from build123d import *

# Parameters (mm, degrees)
SKETCH1_R           = 1.5
BOSS_EXTRUDE1_DEPTH = 5


with BuildPart() as part:
    # Sketch1 → Boss-Extrude1 (new body)
    with BuildSketch(Plane(origin=(0, 0, 0), x_dir=(1, 0, 0), z_dir=(0, 1, 0))):
        with BuildLine():
            Line((12.5, -22.5), (-12.5, -22.5))
            ThreePointArc((-12.5, -22.5), (-19.571067812, -19.571067812), (-22.5, -12.5))
            Line((-22.5, -12.5), (-22.5, 12.5))
            ThreePointArc((-22.5, 12.5), (-19.571067812, 19.571067812), (-12.5, 22.5))
            Line((-12.5, 22.5), (12.5, 22.5))
            ThreePointArc((12.5, 22.5), (19.571067812, 19.571067812), (22.5, 12.5))
            Line((22.5, 12.5), (22.5, -12.5))
            ThreePointArc((22.5, -12.5), (19.571067812, -19.571067812), (12.5, -22.5))
        make_face()
        with Locations(Location((-15, 15, 0), (0, 0, 270))):
            Circle(SKETCH1_R, mode=Mode.SUBTRACT)
        with Locations(Location((15, 15, 0), (0, 0, 90))):
            Circle(SKETCH1_R, mode=Mode.SUBTRACT)
        with Locations(Location((15, -15, 0), (0, 0, 270))):
            Circle(SKETCH1_R, mode=Mode.SUBTRACT)
        with Locations(Location((-15, -15, 0), (0, 0, 90))):
            Circle(SKETCH1_R, mode=Mode.SUBTRACT)
    extrude(amount=BOSS_EXTRUDE1_DEPTH)

    # Sketch5 → Revolve5 (revolve)
    with BuildSketch(Plane.XY, mode=Mode.PRIVATE) as revolve5_sk:
        with BuildLine():
            Line((0, 0), (0, -30))
            Line((0, -30), (-14.490872109, -30))
            ThreePointArc((-14.490872109, -30), (-10.310219401, -15), (-14.490872109, 0))
            Line((-14.490872109, 0), (0, 0))
        make_face()
    revolve(revolve5_sk.sketch.rotate(Axis((0, 6.623218914, 0), (0, -1, 0)), 270), axis=Axis((0, 6.623218914, 0), (0, -1, 0)))

    # Sketch6 → Revolve6 (revolve)
    with BuildSketch(Plane(origin=(0, 0, 0), x_dir=(0, 0, -1), z_dir=(1, 0, 0))):
        with BuildLine():
            Line((0, -17.323751058), (0, -59.119175033))
            ThreePointArc((0, -59.119175033), (-20.897711988, -38.221463045), (0, -17.323751058))
        make_face()
    revolve(axis=Axis((0, -62.962580504, 0), (0, 1, 0)))


solid = part.part
CAD build for the part. Positions are in the model's coordinates, mm. A direction names the side the tool comes from. Round coordinates to 2 decimals unless told otherwise and drop trailing zeros. Write each loop counter-clockwise with the first axis right and the second up, starting at its lowest first coordinate (ties: lowest second). Pieces come first, ordered by that corner, then holes. Notation, with made-up numbers: M 29.25,69.25 L 62.25,69.25 A21 ccw 62.25,98.25 Z; hole C -0.5,24.5 d9. An arc over 180 degrees is marked long. Use a Markdown table: item, result. Add a question column.
1. Flat gauge pins, fed straight in: P1, Ø10, axis at y = -45, z = 1, coming from the +X side; P2, Ø12, axis at y = -31, z = -15.5, coming from the -X side; P3, Ø6, axis at x = 1, z = -8, coming from the -Y side. Where does each tip first touch, or does it go through?
2. Pull direction X, two halves, no side cores. Call faces 4 (the face through (14.93, 2.46, -13.5)), 5 (the face through (19.65, 2.46, 19.49)), 6 (the face through (-19.65, 2.46, -19.49)), 7 (the face through (-15.07, 2.46, 16.5)): released by +X, released by -X, zero draft, split by the parting line, or undercut.
3. Slice it at B-B on y = -49.5. Give the cut face in (x, z).
4. Slice it at A-A on y = -15.5. Give the cut face in (x, z), then the cut area to 3 significant figures.
5. 3-axis set-ups, long thin cutter, end or side, ignore diameter. For faces 1 (the face through (0, 2, 22.5)), 2 (the face through (0, 0, -15)), 3 (the face through (15.07, 2.46, 13.5)): which of +Z, -Z, +X, -X, +Y, -Y reach the whole face in a straight line?
6. Drill centre lines: probe 1 along X at (y, z) = (2, -15); probe 2 along Y at (x, z) = (16, -16.5); probe 3 along Y at (x, z) = (16.5, 3). Where is each one in solid material? Low to high.
Reply:
| question | item | result |
|---|---|---|
| 1 | P1 | stops at x = 20.82 |
| 1 | P2 | stops at x = -17.71 |
| 1 | P3 | stops at y = -58.5 |
| 2 | face 4 | undercut |
| 2 | face 5 | released by +X |
| 2 | face 6 | released by -X |
| 2 | face 7 | undercut |
| 3 | outline | C 0,0 d35.19 |
| 4 | outline | C 0,0 d20.63 |
| 4 | area | 334 mm^2 |
| 5 | face 1 | +Z, +X, -X, +Y, -Y |
| 5 | face 2 | none |
| 5 | face 3 | +Y |
| 6 | probe 1 | x = -22.18 to -16.5, -13.5 to 13.5, 16.5 to 22.18 |
| 6 | probe 2 | y = 0 to 5 |
| 6 | probe 3 | y = -50.69 to -25.75, 0 to 5 |
